The listing builds one solid part. Answer for the finished solid, in the listing's coordinates (mm). Coordinates: 2 decimals unless noted, no trailing zeros. Write each loop counter-clockwise with the first axis right and the second up, starting at its lowest first coordinate (ties: lowest second). Pieces come first, ordered by that corner, then holes. Notation, with made-up numbers: M 77,-9.75 L 89,-9.75 A17 cw 89,14.25 Z; hole C 25.5,55 d9. An arc over 180 degrees is marked long. Answer as CSV lines item,"result". Start each with the question number.
```python
from build123d import *

# Parameters (mm, degrees)
SKETCH1_W           = 165
SKETCH1_H           = 110
BOSS_EXTRUDE1_DEPTH = 6
SKETCH2_W           = 5
SKETCH2_H           = 35
SKETCH2_W_2         = 74
SKETCH2_H_2         = 5
SKETCH2_W_3         = 2.2
SKETCH2_H_3         = 10.2
CUT_EXTRUDE1_DEPTH  = 3
SKETCH3_R           = 1.5
CUT_EXTRUDE2_DEPTH  = 111.956279878


with BuildPart() as part:
    # Sketch1 → Boss-Extrude1 (new body)
    with BuildSketch(Plane(origin=(0, 0, 0), x_dir=(1, 0, 0), z_dir=(0, 1, 0))):
        with Locations((-12.658730159, 1.746031746)):
            Rectangle(SKETCH1_W, SKETCH1_H)
    extrude(amount=BOSS_EXTRUDE1_DEPTH)

    # Sketch2 → Cut-Extrude1 (cut)
    with BuildSketch(Plane(origin=(0, 6, 0), x_dir=(1, 0, 0), z_dir=(0, 1, 0))):
        Polygon((-92.658730159, 48.746031746), (-92.658730159, 35.746031746), (-87.658730159, 35.746031746), (-87.658730159, 43.746031746), (-79.658730159, 43.746031746), (-79.658730159, 48.746031746), align=None)
        Polygon((-79.658730159, -40.253968254), (-79.658730159, -45.253968254), (-92.658730159, -45.253968254), (-92.658730159, -32.253968254), (-87.658730159, -32.253968254), (-87.658730159, -40.253968254), align=None)
        Polygon((54.341269841, 43.746031746), (54.341269841, 48.746031746), (67.341269841, 48.746031746), (67.341269841, 35.746031746), (62.341269841, 35.746031746), (62.341269841, 43.746031746), align=None)
        Polygon((62.341269841, -40.253968254), (54.341269841, -40.253968254), (54.341269841, -45.253968254), (67.341269841, -45.253968254), (67.341269841, -32.253968254), (62.341269841, -32.253968254), align=None)
        with Locations((64.841269841, 1.746031746)):
            Rectangle(SKETCH2_W, SKETCH2_H)
        with Locations((-90.158730159, 1.746031746)):
            Rectangle(SKETCH2_W, SKETCH2_H)
        with Locations((-12.658730159, -42.753968254)):
            Rectangle(SKETCH2_W_2, SKETCH2_H_2)
        with Locations((-12.658730159, 46.246031746)):
            Rectangle(SKETCH2_W_2, SKETCH2_H_2)
        with Locations((-77.408730159, 46.966237914)):
            Rectangle(SKETCH2_W_3, SKETCH2_H_3)
        with Locations((-62.908730159, 46.966237914)):
            Rectangle(SKETCH2_W_3, SKETCH2_H_3)
        with Locations((52.091269841, 46.966237914)):
            Rectangle(SKETCH2_W_3, SKETCH2_H_3)
        with Locations((37.591269841, 46.966237914)):
            Rectangle(SKETCH2_W_3, SKETCH2_H_3)
        with Locations((52.091269841, -43.474174422)):
            Rectangle(SKETCH2_W_3, SKETCH2_H_3)
        with Locations((37.591269841, -43.474174422)):
            Rectangle(SKETCH2_W_3, SKETCH2_H_3)
        with Locations((-62.908730159, -43.474174422)):
            Rectangle(SKETCH2_W_3, SKETCH2_H_3)
        with Locations((-77.408730159, -43.474174422)):
            Rectangle(SKETCH2_W_3, SKETCH2_H_3)
    extrude(amount=-CUT_EXTRUDE1_DEPTH, mode=Mode.SUBTRACT)

    # Sketch3 → Cut-Extrude2 (cut, through all)
    with BuildSketch(Plane(origin=(0, 6, 0), x_dir=(1, 0, 0), z_dir=(0, 1, 0))):
        with Locations(Location((-37.658730159, 51.246031746, 0), (0, 0, 270))):
            Circle(SKETCH3_R)
        with Locations(Location((12.341269841, 51.246031746, 0), (0, 0, 90))):
            Circle(SKETCH3_R)
        with Locations(Location((-12.658730159, 51.246031746, 0), (0, 0, 270))):
            Circle(SKETCH3_R)
        with Locations(Location((12.341269841, -47.753968254, 0), (0, 0, 270))):
            Circle(SKETCH3_R)
        with Locations(Location((-12.658730159, -47.753968254, 0), (0, 0, 90))):
            Circle(SKETCH3_R)
        with Locations(Location((-37.658730159, -47.753968254, 0), (0, 0, 90))):
            Circle(SKETCH3_R)
    extrude(amount=-CUT_EXTRUDE2_DEPTH, mode=Mode.SUBTRACT)


solid = part.part
```
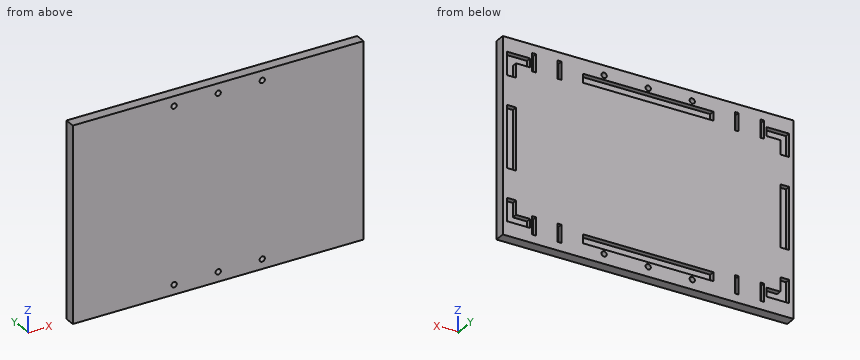
1) Find the intervals of material crossed by line 1 (Z direction, x = 57.5, y = 3.8); line 2 (X direction, y = 5.7, z = 6); line 3 (Y direction, x = -24.5, z = 43.5), in increasing order. Write a range as from..to.
2) The part is cut by section C-C (y = 4.85). Count the separate pieces of the cut face and the enclosed holes in it, then the cut area to 3 significant figures.
3) The part is cut by section B-B (z = -38). Determine the outline of the cut face in (x, y).
4) Each of these flat-tipped pins is pushed along its axis until it touches: P1, Ø12, axis at x = 3, z = -39.5, coming from the -Y side; P2, Ø1.1, axis at x = -62.5, z = -45, coming from the +Y side. Where does it stop, or does it pass through?
5) The part is cut by section A-A (x = 18). Determine the outline of the cut face in (y, z).
Completed:
1,line 1,"-56.75..-48.75, -43.75..40.25, 45.25..53.25"
1,line 2,"-95.16..-92.66, -87.66..62.34, 67.34..69.84"
1,line 3,"0..3"
2,separate pieces,"1"
2,enclosed holes,"22"
2,area,"16,400 mm²"
3,outline,"M -95.16,0 L 69.84,0 L 69.84,6 L 67.34,6 L 67.34,3 L 62.34,3 L 62.34,6 L -87.66,6 L -87.66,3 L -92.66,3 L -92.66,6 L -95.16,6 Z"
4,P1,"y = 0"
4,P2,"y = 3"
5,outline,"M 0,-56.75 L 6,-56.75 L 6,-48.75 L 3,-48.75 L 3,-43.75 L 6,-43.75 L 6,40.25 L 3,40.25 L 3,45.25 L 6,45.25 L 6,53.25 L 0,53.25 Z"
